```python
from build123d import *

# Parameters (mm, degrees)
SKETCH4_W                  = 106
SKETCH4_H                  = 30
BOSS_EXTRUDE2_DEPTH        = 13
SKETCH25_W                 = 106
SKETCH25_H                 = 8.1
CUT_EXTRUDE3_DEPTH         = 1
CUT_EXTRUDE3_DEPTH_BACK    = 8.3
M3X0_5_TAPPED_HOLE1_D      = 2.5
SKETCH28_W                 = 106
SKETCH28_H                 = 4.5
BOSS_EXTRUDE3_DEPTH        = 41.5
SKETCH32_W                 = 41.5
SKETCH32_H                 = 4.5
BOSS_EXTRUDE10_DEPTH       = 5
SKETCH33_W                 = 13
SKETCH33_H                 = 17.621445937
BOSS_EXTRUDE12_DEPTH       = 5
SKETCH34_W                 = 4.498886861
SKETCH34_H                 = 13.121445937
BOSS_EXTRUDE13_DEPTH       = 7
SKETCH35_W                 = 54.5
SKETCH35_H                 = 4.5
BOSS_EXTRUDE14_DEPTH       = 40
SKETCH36_W                 = 5
SKETCH36_H                 = 20
BOSS_EXTRUDE15_DEPTH       = 13.12
F_8_0_199_DIAMETER_HOLE1_D = 5.0546
SKETCH39_R                 = 7
CUT_EXTRUDE4_DEPTH         = 10
M2_CLEARANCE_HOLE1_D       = 2.4
M5_CLEARANCE_HOLE1_D       = 5.5
SKETCH43_W                 = 35.304815243
SKETCH43_H                 = 4
BOSS_EXTRUDE16_DEPTH       = 70


with BuildPart() as part:
    # Sketch4 → Boss-Extrude2 (new body)
    with BuildSketch(Plane.XY):
        with Locations((-36.891047602, -35.322762913)):
            Rectangle(SKETCH4_W, SKETCH4_H)
    extrude(amount=-BOSS_EXTRUDE2_DEPTH)

    # Sketch25 → Cut-Extrude3 (cut, two sides)
    with BuildSketch(Plane.XY) as cut_extrude3_sk:
        with Locations((-36.891047602, -28.651316976)):
            Rectangle(SKETCH25_W, SKETCH25_H)
    extrude(amount=CUT_EXTRUDE3_DEPTH, mode=Mode.SUBTRACT)
    extrude(cut_extrude3_sk.sketch, amount=-CUT_EXTRUDE3_DEPTH_BACK, mode=Mode.SUBTRACT)

    # M3x0.5 Tapped Hole1 (through all)
    with Locations(Plane(origin=(-74.390985602, -20.322762913, -4.15), x_dir=(0, 0, 1), z_dir=(0, 1, 0))):
        with Locations((0, 0), (0, 25), (-0.055677319, 74.999938), (0, 50)):
            Hole(M3X0_5_TAPPED_HOLE1_D / 2)

    # Sketch28 → Boss-Extrude3 (add)
    with BuildSketch(Plane.XY):
        with Locations((-36.891047602, -48.072762913)):
            Rectangle(SKETCH28_W, SKETCH28_H)
    extrude(amount=BOSS_EXTRUDE3_DEPTH)

    # Sketch32 → Boss-Extrude10 (add)
    with BuildSketch(Plane.ZY.offset(89.891047602)):
        with Locations((20.75, -48.072762913)):
            Rectangle(SKETCH32_W, SKETCH32_H)
    extrude(amount=BOSS_EXTRUDE10_DEPTH)

    # Sketch33 → Boss-Extrude12 (add)
    with BuildSketch(Plane.ZY.offset(89.891047602)):
        with Locations((-6.5, -41.512039945)):
            Rectangle(SKETCH33_W, SKETCH33_H)
    extrude(amount=BOSS_EXTRUDE12_DEPTH)

    # Sketch34 → Boss-Extrude13 (add)
    with BuildSketch(Plane.XY):
        with Locations((-92.641604172, -39.262039945)):
            Rectangle(SKETCH34_W, SKETCH34_H)
    extrude(amount=BOSS_EXTRUDE13_DEPTH)

    # Sketch35 → Boss-Extrude14 (add)
    with BuildSketch(Plane.ZY.offset(94.891047602)):
        with Locations((14.25, -48.072762913)):
            Rectangle(SKETCH35_W, SKETCH35_H)
    extrude(amount=BOSS_EXTRUDE14_DEPTH)

    # Sketch36 → Boss-Extrude15 (add)
    with BuildSketch(Plane(origin=(0, -45.822762913, 0), x_dir=(1, 0, 0), z_dir=(0, 1, 0))):
        with Locations((-93.41812931, -31.5)):
            Rectangle(SKETCH36_W, SKETCH36_H)
    extrude(amount=BOSS_EXTRUDE15_DEPTH)

    # #8 (0.199) Diameter Hole1 (through all)
    with Locations(Plane(origin=(-80.669073904, -45.822762913, 14.25), x_dir=(0, 0, 1), z_dir=(0, 1, 0))):
        with Locations((0, 0), (0, 91.778026302), (0, 81.778026302), (0, 10)):
            Hole(F_8_0_199_DIAMETER_HOLE1_D / 2)

    # Sketch39 → Cut-Extrude4 (cut)
    with BuildSketch(Plane(origin=(0, -45.822762913, 0), x_dir=(1, 0, 0), z_dir=(0, 1, 0))):
        with Locations((-115.41812931, -14.25)):
            Circle(SKETCH39_R)
    extrude(amount=-CUT_EXTRUDE4_DEPTH, mode=Mode.SUBTRACT)

    # M2 Clearance Hole1 (through all)
    with Locations(Plane(origin=(-107.41812931, -45.822762913, 14.25), x_dir=(0, 0, 1), z_dir=(0, 1, 0))):
        with Locations((0, 0), (8.000007036, -8.002918292), (-7.999992964, -8.002918292), (0, -16)):
            Hole(M2_CLEARANCE_HOLE1_D / 2)

    # M5 Clearance Hole1 (through all)
    with Locations(Plane(origin=(0.608952398, -50.322762913, 33), x_dir=(0, 0, -1), z_dir=(0, -1, 0))):
        with Locations((0, 0), (0, -25), (0, -50), (0, -75)):
            Hole(M5_CLEARANCE_HOLE1_D / 2)

    # Sketch43 → Boss-Extrude16 (add)
    with BuildSketch(Plane(origin=(0, -50.322762913, 0), x_dir=(-1, 0, 0), z_dir=(0, -1, 0))):
        Polygon((95.586232359, -37.5), (95.586232359, -41.5), (134.891047602, -41.5), (134.891047602, -37.5), (130.891047602, -37.5), align=None)
        Polygon((130.891047602, -37.5), (134.891047602, -37.5), (134.891047602, 13), (130.891047602, 13), (130.891047602, 9), align=None)
        with Locations((113.238639981, 11)):
            Rectangle(SKETCH43_W, SKETCH43_H)
    extrude(amount=BOSS_EXTRUDE16_DEPTH)


solid = part.part
```
Build history of the part. All positions in model axes, mm. A direction names the side the tool comes from. Give positions to 0.01 mm unless a question says otherwise; leave off trailing zeros. Loops run counter-clockwise (first coordinate to the right, second up) from the corner with the lowest first, then second, coordinate; pieces in that order, holes last.
Item 1: Flat gauge pins, fed straight in: pin 1 (4 mm diameter, centred on x = -123.42, z = 14.25, fed in from -Y); pin 2 (1 mm diameter, centred on y = -65.5, z = 29.5, fed in from +X); pin 3 (7 mm diameter, centred on x = -49.39, z = 33, fed in from +Y). Where does each tip first touch, or does it go through?
Answers follow:
pin 1: stops at y = -50.32
pin 2: stops at x = -130.89
pin 3: stops at y = -45.82
Item 2: Slice it at D-D, the plane y = -70. List the corners of the cut face in (x, z).
Answers follow:
outline: (-134.89, -13) - (-95.59, -13) - (-95.59, -9) - (-130.89, -9) - (-130.89, 37.5) - (-95.59, 37.5) - (-95.59, 41.5) - (-134.89, 41.5) - close
Item 3: Slice it at C-C, the plane y = -43.5. List the corners of the cut face in (x, z).
Answers follow:
outline: (-95.92, 21.5) - (-90.92, 21.5) - (-90.92, 41.5) - (-95.92, 41.5) - close; (-94.89, -13) - (16.11, -13) - (16.11, 0) - (-90.39, 0) - (-90.39, 7) - (-94.89, 7) - close; hole circle Ø2.5 at (-74.39, -4.15); hole circle Ø2.5 at (-49.39, -4.15); hole circle Ø2.5 at (-24.39, -4.15); hole circle Ø2.5 at (0.61, -4.21)
Item 4: Which spindle directions (+Z, -Z, +X, -X, +Y, -Y) get a long thin tool onto all of the face, cutting with end or side? Do faces 1 (the face through (-95.586, -85, -11)), 2 (the face through (-94.891, -39, -3)), 3 (the face through (-90.918, -39, 32)), 4 (the face through (-130.891, -85, 14)). Say none if no direction does.
Answers follow:
face 1: +Z, -Z, +X, -Y
face 2: -Z, -X, +Y
face 3: +Z, +X, +Y
face 4: +X, -Y
Item 5: Slice it at A-A, the plane z = 33. List the corners of the cut face in (x, y), and give its area (3 significant figures).
Answers follow:
outline: (-134.89, -120.32) - (-130.89, -120.32) - (-130.89, -50.32) - (-77.14, -50.32) - (-77.14, -45.82) - (-90.92, -45.82) - (-90.92, -32.7) - (-95.92, -32.7) - (-95.92, -45.82) - (-134.89, -45.82) - close; (-71.64, -50.32) - (-52.14, -50.32) - (-52.14, -45.82) - (-71.64, -45.82) - close; (-46.64, -50.32) - (-27.14, -50.32) - (-27.14, -45.82) - (-46.64, -45.82) - close; (-21.64, -50.32) - (-2.14, -50.32) - (-2.14, -45.82) - (-21.64, -45.82) - close; (3.36, -50.32) - (16.11, -50.32) - (16.11, -45.82) - (3.36, -45.82) - close
area: 926 mm2
Item 6: Drill centre lines: line 1 (X direction, y = -48.25, z = 14.25); line 2 (X direction, y = -47, z = 33); line 3 (Z direction, x = -115, y = -67). Where is each one in solid material? Low to high.
Answers follow:
line 1: x = -134.89 to -124.62, -106.22 to -83.2, -78.14 to -73.2, -68.14 to -1.42, 3.64 to 8.58, 13.64 to 16.11
line 2: x = -134.89 to -77.14, -71.64 to -52.14, -46.64 to -27.14, -21.64 to -2.14, 3.36 to 16.11
line 3: z = -13 to -9, 37.5 to 41.5
Item 7: Slice it at B-B, the plane x = -10.5. List the corners of the cut face in (y, z).
Answers follow:
outline: (-50.32, -13) - (-20.32, -13) - (-20.32, 0) - (-24.6, 0) - (-24.6, -8.3) - (-32.7, -8.3) - (-32.7, 0) - (-45.82, 0) - (-45.82, 41.5) - (-50.32, 41.5) - close
Item 8: Pull direction Y, two halves, no side cores. Call faces 5 (the face through (-93, -32.703, 31)), 6 (the face through (-38, -29, -8.3)), 7 (the face through (-40, -32.701, -3)), 8 (the face through (-104, -80, 41.5)): released by +Y, released by -Y, zero draft, split by the parting line, or undercut.
Answers follow:
face 5: released by +Y
face 6: undercut
face 7: undercut
face 8: zero draft
